```python
from build123d import *

# Parameters (mm, degrees)
PAD_DEPTH = 1
FILLET_R  = 5


with BuildPart() as part:
    # Sketch → Pad (new body)
    with BuildSketch(Plane.XY):
        with BuildLine():
            Line((-105, 0), (105, 0))
            Line((105, 0), (105, 175))
            ThreePointArc((105, 175), (0, 200), (-105, 175))
            Line((-105, 0), (-105, 175))
        make_face()
    extrude(amount=PAD_DEPTH)

    # Fillet
    fillet_edges = [part.edges().sort_by_distance(p)[0] for p in [
        (105, 0, 0.5),
        (105, 175, 0.5),
        (-105, 175, 0.5),
        (-105, 0, 0.5),
    ]]
    fillet(fillet_edges, radius=FILLET_R)


solid = part.part
```
Input: part model. Units: mm. Frame: model coordinates. Give positions to 0.01 mm unless a question says otherwise; leave off trailing zeros. Order: outer loops, then holes, each group sorted by start corner. A loop starts at its lowest first (then second) coordinate and runs counter-clockwise, first axis right, second up. Notation, with made-up numbers: M 20.5,10 L 78.5,10 A17 cw 78.5,14 Z; hole C 71,63 d8. An arc over 180 degrees is marked long. One line per question, with ' | ' between items. Start each with the question number.
1. Section query A-A (z = 0.4). Return the cut outline in (x, y).
2. Material intervals for probe 1 along Y at (x, z) = (23.5, 0.1); probe 2 along Y at (x, z) = (38.5, 0.7), sorted ascending. Write a range as [from, to].
3. Section query B-B (x = -83). Return the cut outline in (y, z).
4. Section query C-C (x = -39.5). Return the cut outline in (y, z), and give its area (3 significant figures).
Here are the results:
1) outline: M -105,5 A5 ccw -100,0 L 100,0 A5 ccw 105,5 L 105,171.9 A5 ccw 102.19,176.39 A233 ccw -102.19,176.39 A5 ccw -105,171.9 Z
2) probe 1: [0, 198.81] | probe 2: [0, 196.8]
3) outline: M 0,0 L 184.72,0 L 184.72,1 L 0,1 Z
4) outline: M 0,0 L 196.63,0 L 196.63,1 L 0,1 Z | area: 197 mm²
